```python
from build123d import *

# Parameters (mm, degrees)
SKETCH1_R           = 20.066
BOSS_EXTRUDE1_DEPTH = 12.7
SKETCH2_R           = 5.461
CUT_EXTRUDE1_DEPTH  = 13.7
BOSS_EXTRUDE2_DEPTH = 12.7


with BuildPart() as part:
    # Sketch1 → Boss-Extrude1 (new body)
    with BuildSketch(Plane.XY):
        Circle(SKETCH1_R)
    extrude(amount=BOSS_EXTRUDE1_DEPTH)

    # Sketch2 → Cut-Extrude1 (cut, through all)
    with BuildSketch(Plane(origin=(0, 0, 0), x_dir=(-1, 0, 0), z_dir=(0, 0, -1))):
        Circle(SKETCH2_R)
    extrude(amount=-CUT_EXTRUDE1_DEPTH, mode=Mode.SUBTRACT)

    # Sketch3 → Boss-Extrude2 (add)
    with BuildSketch(Plane(origin=(0, 0, 0), x_dir=(-1, 0, 0), z_dir=(0, 0, -1))):
        with BuildLine():
            Line((-19.117613345, -6.096), (-14.9225, 0))
            Line((-14.9225, 0), (-19.117613345, 6.096))
            ThreePointArc((-19.117613345, 6.096), (-20.066, 0), (-19.117613345, -6.096))
        make_face()
        with BuildLine():
            Line((19.117613345, 6.096), (14.9225, 0))
            Line((14.9225, 0), (19.117613345, -6.096))
            ThreePointArc((19.117613345, -6.096), (20.066, 0), (19.117613345, 6.096))
        make_face()
        with BuildLine():
            Line((0, 18.415), (-4.3815, 10.27697427))
            Line((-4.3815, 10.27697427), (-1.651, 5.205450989))
            ThreePointArc((-1.651, 5.205450989), (0, 5.461), (1.651, 5.205450989))
            Line((1.651, 5.205450989), (4.3815, 10.27697427))
            Line((4.3815, 10.27697427), (0, 18.415))
        make_face()
        with BuildLine():
            Line((-1.651, -5.205450989), (-4.3815, -10.27697427))
            Line((-4.3815, -10.27697427), (0, -18.415))
            Line((0, -18.415), (4.3815, -10.27697427))
            Line((4.3815, -10.27697427), (1.651, -5.205450989))
            ThreePointArc((1.651, -5.205450989), (0, -5.461), (-1.651, -5.205450989))
        make_face()
    extrude(amount=BOSS_EXTRUDE2_DEPTH)


solid = part.part
```
Check sheet for the modelled part. Datum: model origin and axes. Units: mm. A direction names the side the tool comes from. Round coordinates to 2 decimals unless told otherwise and drop trailing zeros. Loops run counter-clockwise (first coordinate to the right, second up) from the corner with the lowest first, then second, coordinate; pieces in that order, holes last. Notation, with made-up numbers: M 24.25,22.5 L 40.25,22.5 A18 cw 40.25,49.5 Z; hole C -12.5,11 d1. An arc over 180 degrees is marked long. Answer as a JSON object with one key per item and string values.
1. Scan lines: line 1 (Y direction, x = 0, z = 8); line 2 (Z direction, x = -16, y = -7). Record each from-to range of solid material in increasing order.
Reply:
{"line 1": "y = -20.07 to -5.46, 5.46 to 20.07", "line 2": "z = 0 to 12.7"}
2. Section check B-B (x = -1). Record the boundary of the cut face in (y, z), plus the area to 3 significant figures.
Reply:
{"outline": "M -20.04,0 L -16.56,0 L -16.56,-12.7 L -5.37,-12.7 L -5.37,12.7 L -20.04,12.7 Z; M 5.37,-12.7 L 16.56,-12.7 L 16.56,0 L 20.04,0 L 20.04,12.7 L 5.37,12.7 Z", "area": "657 mm²"}
3. Gauge pin test, flat ends, axial feed: P1, Ø6, axis at y = 11.5, z = -7, coming from the +X side; P2, Ø3, axis at x = 14, z = 6, coming from the -Y side; P3, Ø8, axis at x = -10.5, y = 9, coming from the -Z side. Record the tip position at first contact, or that the pin passes through.
Reply:
{"P1": "stops at x = 4.38", "P2": "stops at y = -15.7", "P3": "stops at z = 0"}
4. Section check D-D (z = 7.25). Record the boundary of the cut face in (x, y), plus the area to 3 significant figures.
Reply:
{"outline": "C 0,0 d40.13; hole C 0,0 d10.92", "area": "1,170 mm²"}
5. Access from +Z, -Z, +X, -X, +Y, -Y to the whole of each face (thin tool, end or side, straight path). Record for faces 1 (the flat face through (-2.22, 14.29, -6.26)), 2 (the flat face through (17.05, -3.09, -6.26)), 3 (the flat face through (2.22, -14.29, -6.26)), 4 (the flat face through (-17.05, 3.09, -6.26)), 5 (the flat face through (3.035, 7.777, -6.261)).
Reply:
{"face 1": "-Z, -X, +Y", "face 2": "-Z, -Y", "face 3": "-Z, +X, -Y", "face 4": "-Z, +Y", "face 5": "-Z"}
6. Section check A-A (z = -2.5). Record the boundary of the cut face in (x, y) (1 decimal).
Reply:
{"outline": "M -19.1,-6.1 L -14.9,0 L -19.1,6.1 A20.1 ccw Z; M -4.4,-10.3 L 0,-18.4 L 4.4,-10.3 L 1.7,-5.2 A5.5 cw -1.7,-5.2 Z; M -4.4,10.3 L -1.7,5.2 A5.5 cw 1.7,5.2 L 4.4,10.3 L 0,18.4 Z; M 14.9,0 L 19.1,-6.1 A20.1 ccw 19.1,6.1 Z"}
7. Section check C-C (y = -8). Record the boundary of the cut face in (x, z), plus the area to 3 significant figures.
Reply:
{"outline": "M -18.4,0 L -3.16,0 L -3.16,-12.7 L 3.16,-12.7 L 3.16,0 L 18.4,0 L 18.4,12.7 L -18.4,12.7 Z", "area": "548 mm²"}
